Check sheet for the drawn part. Datum: minimum x, y, z corner. Units: mm. A direction names the side the tool comes from. Round coordinates to 2 decimals unless told otherwise and drop trailing zeros. Loops run counter-clockwise (first coordinate to the right, second up) from the corner with the lowest first, then second, coordinate; pieces in that order, holes last.
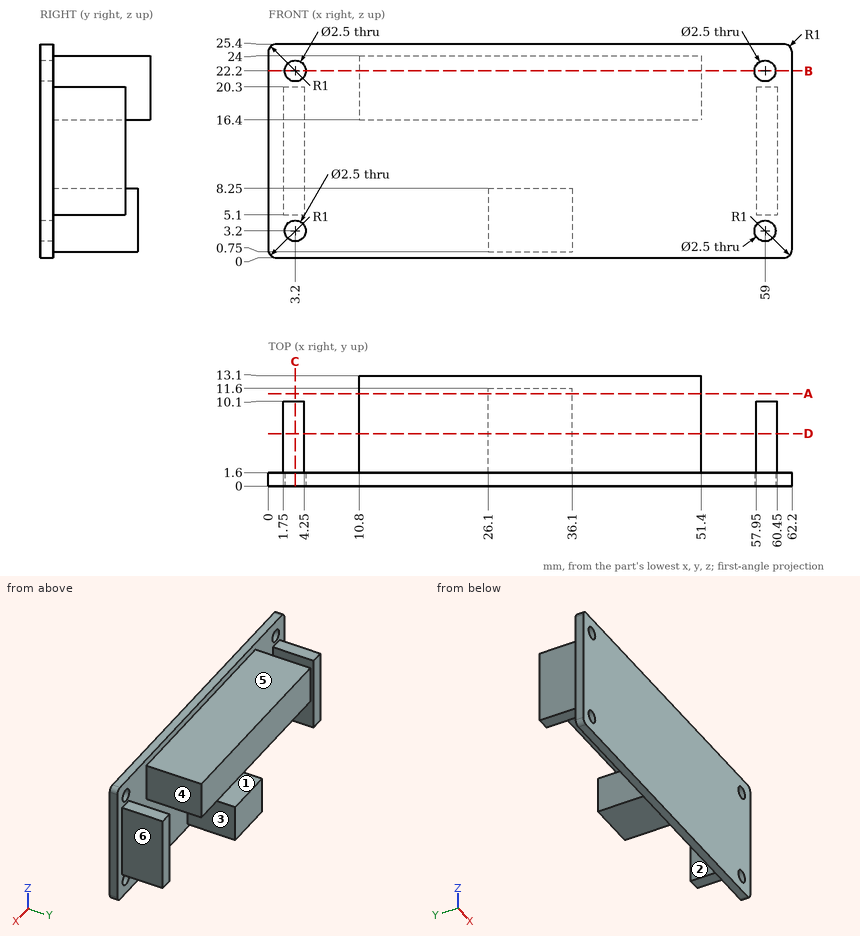
1. Scan lines: L1, parallel to X at y = 0.75, z = 22.2; L2, parallel to X at y = 2.25, z = 19; L3, parallel to X at y = 3.5, z = 12.25. Record each from-to range of solid material in increasing order.
2. Tool access check on the marked faces 1, 2 and 3. Record the directions out of +Z, -Z, +X, -X, +Y, -Y that give a thin tool (end or side, any length) a straight path to the whole face; none if there is none.
3. Section check D-D (y = 6.25). Enter the section's corners in (x, z).
4. Section check A-A (y = 11). Enter the section's corners in (x, z).
5. Release check for a two-part mould opening along X. For the marked faces 4, 5 and 6 record: released by +X, released by -X, zero draft, split by the parting line, or undercut.
6. Gauge pin test, flat ends, axial feed: P1, Ø2, axis at y = 8.5, z = 18.5, coming from the +X side; P2, Ø2, axis at x = 30, z = 3, coming from the +Y side; P3, Ø3, axis at y = 5, z = 10, coming from the -X side; P4, Ø2, axis at x = 59, z = 22.2, coming from the -Y side. Record the tip position at first contact, or that the pin passes through.
7. Section check C-C (x = 3.2). Enter the section's corners in (y, z), then the cut area to 3 significant figures.
8. Section check B-B (z = 22.2). Enter the section's corners in (x, y), then the cut area to 3 significant figures.
Taken from the geometry:
1. L1: x = 0 to 1.95, 4.45 to 57.75, 60.25 to 62.2
1. L2: x = 1.75 to 4.25, 10.8 to 51.4, 57.95 to 60.45
1. L3: x = 1.75 to 4.25, 57.95 to 60.45
2. face 1: +Y
2. face 2: +Z, -Z, +Y
2. face 3: -Z, +Y
3. outline: (1.75, 5.1) - (4.25, 5.1) - (4.25, 20.3) - (1.75, 20.3) - close; (10.8, 16.4) - (51.4, 16.4) - (51.4, 24) - (10.8, 24) - close; (26.1, 0.75) - (36.1, 0.75) - (36.1, 8.25) - (26.1, 8.25) - close; (57.95, 5.1) - (60.45, 5.1) - (60.45, 20.3) - (57.95, 20.3) - close
4. outline: (10.8, 16.4) - (51.4, 16.4) - (51.4, 24) - (10.8, 24) - close; (26.1, 0.75) - (36.1, 0.75) - (36.1, 8.25) - (26.1, 8.25) - close
5. face 4: undercut
5. face 5: zero draft
5. face 6: released by +X
6. P1: stops at x = 60.45
6. P2: stops at y = 11.6
6. P3: stops at x = 1.75
6. P4: passes through
7. outline: (0, 0) - (1.6, 0) - (1.6, 1.95) - (0, 1.95) - close; (0, 4.45) - (1.6, 4.45) - (1.6, 5.1) - (10.1, 5.1) - (10.1, 20.3) - (1.6, 20.3) - (1.6, 20.95) - (0, 20.95) - close; (0, 23.45) - (1.6, 23.45) - (1.6, 25.4) - (0, 25.4) - close
7. area: 162 mm2
8. outline: (0, 0) - (1.95, 0) - (1.95, 1.6) - (0, 1.6) - close; (4.45, 0) - (57.75, 0) - (57.75, 1.6) - (51.4, 1.6) - (51.4, 13.1) - (10.8, 13.1) - (10.8, 1.6) - (4.45, 1.6) - close; (60.25, 0) - (62.2, 0) - (62.2, 1.6) - (60.25, 1.6) - close
8. area: 558 mm2
